```python
from build123d import *

# Parameters (mm, degrees)
F2_W     = 25.4
F2_H     = 25.4
F3_DEPTH = 12.7


with BuildPart() as f1:
    # F0 (on Front) → F1 (revolve)
    with BuildSketch(Plane.XZ):
        with BuildLine():
            Line((-79.375, 3.175), (-79.375, 5.715))
            ThreePointArc((-79.375, 5.715), (-83.416115, 4.041115), (-85.09, 0))
            Line((-85.09, 0), (0, 0))
            ThreePointArc((0, 0), (-1.673885, 4.041115), (-5.715, 5.715))
            Line((-5.715, 5.715), (-5.715, 3.175))
            Line((-5.715, 3.175), (-79.375, 3.175))
        make_face()
    revolve(axis=Axis((8.346166, 0, 0), (1, 0, 0)))

    # F2 (on Front) → F3 (join, symmetric)
    with BuildSketch(Plane.XZ):
        with Locations((-42.545, 0)):
            Rectangle(F2_W, F2_H)
    extrude(amount=F3_DEPTH, both=True)

    # F5 (on plane+point) → F6 (revolve, cut)
    with BuildSketch(Plane.YZ.offset(-42.545)):
        Polygon((-12.7, 6.0325), (-12.7, 0), (12.7, 0), (12.7, 6.0325), (11.43, 4.7625), (-11.43, 4.7625), align=None)
    revolve(axis=Axis((-42.545, 22.809027, 0), (0, 1, 0)), mode=Mode.SUBTRACT)


solid = f1.part
```
Verification items for the finished model (mm, model axes). A direction names the side the tool comes from. Coordinates: 2 decimals unless noted, no trailing zeros. Loops run counter-clockwise (first coordinate to the right, second up) from the corner with the lowest first, then second, coordinate; pieces in that order, holes last. Notation, with made-up numbers: (-38.75, 31) - (-25.75, 31) arc R23 cw to (-25.75, 68) - close; hole circle Ø3 at (-35.75, 10.25). An arc over 180 degrees is marked (long way). Return JSON: item names as keys, results as strings.
1. Section check A-A, the plane x = -12.5. Record the boundary of the cut face in (y, z) (3 decimals), then the cut area to 3 significant figures.
Established:
{"outline": "circle Ø6.35 at (0, 0)", "area": "31.7 mm2"}
2. Thickness scan on L1, parallel to X at y = -3.5, z = -2.25 (3 decimals); L2, parallel to X at y = 4.75, z = 0 (1 decimal); L3, parallel to X at y = -1.25, z = 8.5 (3 decimals). Record the ranges inside material, lowest first.
Established:
{"L1": "x = -83.293 to -79.375, -55.245 to -46.742, -38.348 to -29.845, -5.715 to -1.797", "L2": "x = -82.6 to -79.4, -55.2 to -47.3, -37.8 to -29.8, -5.7 to -2.5", "L3": "x = -55.245 to -29.845"}
3. Mould release check, pull along Z, two halves, no side actions. Record for faces 3 (the cylindrical face through (-46.77, -0.16, 2.2)), 4 (the flat face through (-29.845, -3, 3)), 5 (the cylindrical face through (-17.95, 3.1, -0.69)): +Z half, -Z half, draft (parallel to the pull), parting line (faces both ways), or undercut.
Established:
{"face 3": "undercut", "face 4": "draft", "face 5": "parting line"}
4. Section check C-C, the plane z = -9. Record the boundary of the cut face in (x, y) (3 decimals), then the cut area to 3 significant figures.
Established:
{"outline": "(-55.245, -12.7) - (-29.845, -12.7) - (-29.845, 12.7) - (-55.245, 12.7) - close", "area": "645 mm2"}
5. Tool access check on faces 1 (the flat face through (-37, -12.7, 3)), 2 (the flat face through (-79.375, 2.5, -2.5)). Record the directions out of +Z, -Z, +X, -X, +Y, -Y that give a thin tool (end or side, any length) a straight path to the whole face; none if there is none.
Established:
{"face 1": "+Z, -Z, +X, -X, -Y", "face 2": "none"}
6. Go/stop test with flat-tipped pins: pin 1 (4 mm diameter, centred on y = -0.5, z = -3.5, fed in from -X); pin 2 (6 mm diameter, centred on y = -7.5, z = 6.5, fed in from +X) (3 decimals); pin 3 (6 mm diameter, centred on y = -2, z = 3, fed in from -X). Record where each tip stops, or that it passes through.
Established:
{"pin 1": "stops at x = -84.88", "pin 2": "stops at x = -29.845", "pin 3": "stops at x = -85.06"}
7. Section check B-B, the plane y = -7.5. Record the boundary of the cut face in (x, z) (1 decimal), then the cut area to 3 significant figures.
Established:
{"outline": "(-55.2, -12.7) - (-29.8, -12.7) - (-29.8, 12.7) - (-55.2, 12.7) - close; hole circle Ø9.5 at (-42.5, 0)", "area": "574 mm2"}
